```python
from build123d import *

# Parameters (mm, degrees)
SKETCH_R        = 54
SKETCH_R_2      = 4.5
SKETCH_R_3      = 2.5
PAD_DEPTH       = 3
SKETCH001_R     = 6.5
SKETCH001_R_2   = 4.5
PAD001_DEPTH    = 7
CHAMFER_SIZE    = 1
SKETCH002_R     = 17
SKETCH002_R_2   = 12.5
PAD002_DEPTH    = 6
CHAMFER001_SIZE = 1


with BuildPart() as part:
    # Sketch → Pad (new body)
    with BuildSketch(Plane.XY):
        Circle(SKETCH_R)
        Circle(SKETCH_R_2, mode=Mode.SUBTRACT)
        with Locations((0, 49)):
            Circle(SKETCH_R_3, mode=Mode.SUBTRACT)
        with Locations((48.25558, 8.508761)):
            Circle(SKETCH_R_3, mode=Mode.SUBTRACT)
        with Locations((42.435245, -24.5)):
            Circle(SKETCH_R_3, mode=Mode.SUBTRACT)
        with Locations((16.758987, -46.044938)):
            Circle(SKETCH_R_3, mode=Mode.SUBTRACT)
        with Locations((-16.758987, -46.044938)):
            Circle(SKETCH_R_3, mode=Mode.SUBTRACT)
        with Locations((-42.435245, -24.5)):
            Circle(SKETCH_R_3, mode=Mode.SUBTRACT)
        with Locations((-48.25558, 8.508761)):
            Circle(SKETCH_R_3, mode=Mode.SUBTRACT)
        with Locations((-31.496593, 37.536178)):
            Circle(SKETCH_R_3, mode=Mode.SUBTRACT)
        with Locations((31.496593, 37.536178)):
            Circle(SKETCH_R_3, mode=Mode.SUBTRACT)
    extrude(amount=PAD_DEPTH)

    # Sketch001 (on Face13 of Pad) → Pad001 (join)
    with BuildSketch(Plane.XY.offset(3)):
        Circle(SKETCH001_R)
        Circle(SKETCH001_R_2, mode=Mode.SUBTRACT)
    extrude(amount=PAD001_DEPTH)

    # Chamfer
    chamfer_edges = [part.edges().sort_by_distance(p)[0] for p in [
        (-6.5, 0, 10),
    ]]
    chamfer(chamfer_edges, length=CHAMFER_SIZE)

    # Sketch002 (on Face3 of Chamfer) → Pad002 (join)
    with BuildSketch(Plane.XY.offset(3)):
        Circle(SKETCH002_R)
        Circle(SKETCH002_R_2, mode=Mode.SUBTRACT)
    extrude(amount=PAD002_DEPTH)

    # Chamfer001
    chamfer001_edges = [part.edges().sort_by_distance(p)[0] for p in [
        (-12.5, 0, 9),
    ]]
    chamfer(chamfer001_edges, length=CHAMFER001_SIZE)


solid = part.part
```
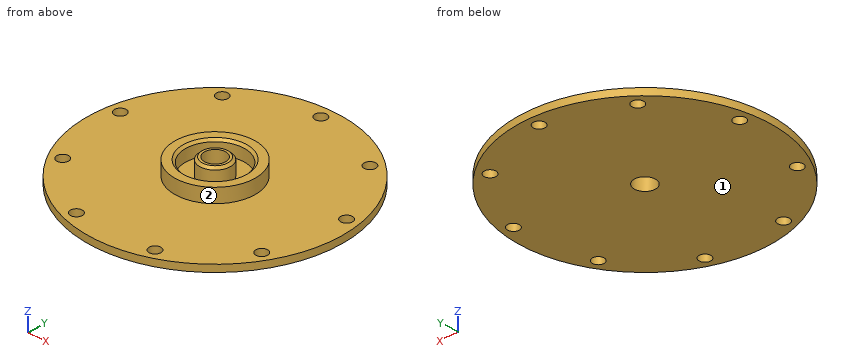
Could you check a few things on this model? Use its own coordinates, in mm. Face numbers are marked on the shaded views. A direction names the side the tool comes from. Give positions to 0.01 mm unless a question says otherwise; leave off trailing zeros. Write each loop counter-clockwise with the first axis right and the second up, starting at its lowest first coordinate (ties: lowest second). Pieces come first, ordered by that corner, then holes. Notation, with made-up numbers: (56, 48.25) - (87, 48.25) arc R20 ccw to (87, 61.25) - close; hole circle Ø5 at (-27.75, 60). An arc over 180 degrees is marked (long way). One line per item, written item: value. Start each with the question number.
Item 1: Imagine slicing it at A-A, the plane x = 0. List the corners of the cut face in (y, z) for me.
Item 2: Please list where these lines run through material, in increasing order: line 1 (Y direction, x = 0, z = 1); line 2 (Y direction, x = 0, z = 5.1); line 3 (Z direction, x = -44, y = -7). Write a range as from..to.
Item 3: Imagine slicing it at B-B, the plane y = 0. List the corners of the cut face in (x, z) for me.
Item 4: Which directions (+Z, -Z, +X, -X, +Y, -Y) give clear straight access to the entire face, cutting with the end or side of a thin tool? Please do the marked faces 1 and 2.
Item 5: Imagine slicing it at C-C, the plane x = 32.5. List the corners of the cut face in (y, z) for me, and give its area (3 significant figures).
Item 6: I'm going to push flat-ended pins straight in: pin 1 (4.5 mm diameter, centred on x = 0, y = 49, fed in from +Z); pin 2 (1 mm diameter, centred on y = 5.5, z = 8, fed in from -X); pin 3 (5 mm diameter, centred on x = 32, y = 8.5, fed in from +Z); pin 4 (4 mm diameter, centred on x = 5, z = 7, fed in from -Y). Where does each tip first touch, or does it pass through?
Item 7: Imagine slicing it at D-D, the plane y = -24.5. List the corners of the cut face in (x, z) for me, and give its area (3 significant figures).
Geometry says:
1. outline: (-54, 0) - (-4.5, 0) - (-4.5, 10) - (-5.5, 10) - (-6.5, 9) - (-6.5, 3) - (-12.5, 3) - (-12.5, 8) - (-13.5, 9) - (-17, 9) - (-17, 3) - (-54, 3) - close; (4.5, 0) - (46.5, 0) - (46.5, 3) - (17, 3) - (17, 9) - (13.5, 9) - (12.5, 8) - (12.5, 3) - (6.5, 3) - (6.5, 9) - (5.5, 10) - (4.5, 10) - close; (51.5, 0) - (54, 0) - (54, 3) - (51.5, 3) - close
2. line 1: -54..-4.5, 4.5..46.5, 51.5..54
2. line 2: -17..-12.5, -6.5..-4.5, 4.5..6.5, 12.5..17
2. line 3: 0..3
3. outline: (-54, 0) - (-4.5, 0) - (-4.5, 10) - (-5.5, 10) - (-6.5, 9) - (-6.5, 3) - (-12.5, 3) - (-12.5, 8) - (-13.5, 9) - (-17, 9) - (-17, 3) - (-54, 3) - close; (4.5, 0) - (54, 0) - (54, 3) - (17, 3) - (17, 9) - (13.5, 9) - (12.5, 8) - (12.5, 3) - (6.5, 3) - (6.5, 9) - (5.5, 10) - (4.5, 10) - close
4. face 1: -Z, +X, -X, +Y, -Y
4. face 2: +Z
5. outline: (-43.12, 0) - (35.25, 0) - (35.25, 3) - (-43.12, 3) - close; (39.83, 0) - (43.12, 0) - (43.12, 3) - (39.83, 3) - close
5. area: 245 mm^2
6. pin 1: through
6. pin 2: x = -16.25
6. pin 3: z = 3
6. pin 4: y = -16.73
7. outline: (-48.12, 0) - (-44.94, 0) - (-44.94, 3) - (-48.12, 3) - close; (-39.94, 0) - (39.94, 0) - (39.94, 3) - (-39.94, 3) - close; (44.94, 0) - (48.12, 0) - (48.12, 3) - (44.94, 3) - close
7. area: 259 mm^2
